```python
from build123d import *

# Parameters (mm, degrees)
SKETCH157_R  = 5
PAD031_DEPTH = 1.4
SKETCH158_W  = 1.8
SKETCH158_H  = 16
PAD032_DEPTH = 6.4
SKETCH159_W  = 1.6
SKETCH159_H  = 4.4
PAD033_DEPTH = 1.4
SKETCH160_W  = 1.4
SKETCH160_H  = 7.4
PAD034_DEPTH = 2.4
PAD035_DEPTH = 1.4


with BuildPart() as part:
    # Sketch157 → Pad031 (new body)
    with BuildSketch(Plane.XY):
        Polygon((1.8, 8), (17, 8), (17, -8), (1.8, -8), (0, -8), (0, 8), align=None)
        with Locations((8.5, 0)):
            Circle(SKETCH157_R, mode=Mode.SUBTRACT)
    extrude(amount=PAD031_DEPTH)

    # Sketch158 (on Face5 of Pad031) → Pad032 (join)
    with BuildSketch(Plane.XY.offset(1.4)):
        with Locations((0.9, 0)):
            Rectangle(SKETCH158_W, SKETCH158_H)
    extrude(amount=PAD032_DEPTH)

    # Sketch159 (on Face6 of Pad032) → Pad033 (join)
    with BuildSketch(Plane.XY.offset(7.8)):
        with Locations((0.9, 0)):
            Rectangle(SKETCH159_W, SKETCH159_H)
    extrude(amount=PAD033_DEPTH)

    # Sketch160 (on Face5 of Pad033) → Pad034 (join)
    with BuildSketch(Plane.XY.offset(1.4)):
        with Locations((16.3, 0)):
            Rectangle(SKETCH160_W, SKETCH160_H)
    extrude(amount=PAD034_DEPTH)

    # Sketch161 (on Face12 of Pad034) → Pad035 (join)
    with BuildSketch(Plane.XY.offset(3.8)):
        Polygon((17, 3.7), (21, 3.7), (21, -3.7), (17, -3.7), (15.6, -3.7), (15.6, 3.7), align=None)
    extrude(amount=PAD035_DEPTH)


solid = part.part
```
For this review, take the finished solid that the model builds, in its own axes (mm). A direction names the side the tool comes from. Round coordinates to 2 decimals unless told otherwise and drop trailing zeros. Write each loop counter-clockwise with the first axis right and the second up, starting at its lowest first coordinate (ties: lowest second). Pieces come first, ordered by that corner, then holes. Notation, with made-up numbers: (20, -2.5) -> (51, -2.5) arc R15 ccw to (51, 3.5) -> close; hole circle Ø10 at (26.5, -17.75). An arc over 180 degrees is marked (long way). Use one line per item in the form item = value.
Q1. Machinability: for faces 1 (the flat face through (1, -2.2, 8)), 2 (the flat face through (18, 0, 5.2)), 3 (the flat face through (17, 0, 1)), 4 (the flat face through (18, 3.7, 4)), which of the approach directions +Z, -Z, +X, -X, +Y, -Y give a long, thin tool a straight path to every point of the face, cutting with its end or side? Answer none if there is none.
Resolved:
face_1 = +Z, +X, -X, -Y
face_2 = +Z, +X, +Y, -Y
face_3 = -Z, +X, +Y, -Y
face_4 = +Z, +X, +Y
Q2. Clearance check with flat-ended pins moving along their axes: pin 1 Ø1.2 at (x, y) = (19.5, 0.5) entering from -Z; pin 2 Ø1.9 at (x, z) = (17, 2.5) entering from -Y; pin 3 Ø6 at (x, y) = (19, -1) entering from +Z. State where each tip first meets the part, or that it passes through.
Resolved:
pin_1 = 3.8
pin_2 = -3.7
pin_3 = 5.2
Q3. The part is to be moulded in two halves that separate along X. For faces 5 (the flat face through (1, 2.2, 8)), 6 (the flat face through (1.8, 0, 5)), 7 (the flat face through (1.7, 0, 8)), say which applies: released by +X, released by -X, zero draft, split by the parting line, or undercut.
Resolved:
face_5 = zero draft
face_6 = undercut
face_7 = released by +X
Q4. Consider section A-A (y = 0). State the section outline as (x, z) points.
Resolved:
outline = (0, 0) -> (3.5, 0) -> (3.5, 1.4) -> (1.8, 1.4) -> (1.8, 7.8) -> (1.7, 7.8) -> (1.7, 9.2) -> (0.1, 9.2) -> (0.1, 7.8) -> (0, 7.8) -> close; (13.5, 0) -> (17, 0) -> (17, 3.8) -> (21, 3.8) -> (21, 5.2) -> (15.6, 5.2) -> (15.6, 1.4) -> (13.5, 1.4) -> close
Q5. To check wall thickness, follow probe 1 along Y at (x, z) = (8.5, 0.35); probe 2 along X at (y, z) = (0, 1.75); probe 3 along Z at (x, y) = (11.25, 7). State the ranges of each line that lie inside material, in increasing order. Write a range as from..to.
Resolved:
probe_1 = -8..-5, 5..8
probe_2 = 0..1.8, 15.6..17
probe_3 = 0..1.4
Q6. Consider section D-D (z = 0.5). State the section outline as (x, y) points, then the cut area to 3 significant figures.
Resolved:
outline = (0, -8) -> (17, -8) -> (17, 8) -> (0, 8) -> close; hole circle Ø10 at (8.5, 0)
area = 193 mm²
Q7. Consider section C-C (x = 8.5). State the section outline as (y, z) points.
Resolved:
outline = (-8, 0) -> (-5, 0) -> (-5, 1.4) -> (-8, 1.4) -> close; (5, 0) -> (8, 0) -> (8, 1.4) -> (5, 1.4) -> close
Q8. Consider section B-B (z = 3). State the section outline as (x, y) points.
Resolved:
outline = (0, -8) -> (1.8, -8) -> (1.8, 8) -> (0, 8) -> close; (15.6, -3.7) -> (17, -3.7) -> (17, 3.7) -> (15.6, 3.7) -> close
